The listing builds one solid part. Answer for the finished solid, in the listing's coordinates (mm). A direction names the side the tool comes from. Give positions to 0.01 mm unless a question says otherwise; leave off trailing zeros. Order: outer loops, then holes, each group sorted by start corner. A loop starts at its lowest first (then second) coordinate and runs counter-clockwise, first axis right, second up. Notation, with made-up numbers: (72.5, 66.25) - (120.5, 66.25) arc R15 ccw to (120.5, 81.25) - close; hole circle Ø6 at (-31, 51). An arc over 180 degrees is marked (long way). Answer in a Markdown table with one row per item.
from build123d import *

# Parameters (mm, degrees)
SKETCH1_R           = 2.5
SKETCH1_R_2         = 1.5
BOSS_EXTRUDE1_DEPTH = 55
SKETCH2_W           = 6
SKETCH2_H           = 1.5
BOSS_EXTRUDE2_DEPTH = 5
SKETCH3_R           = 1
CUT_EXTRUDE1_DEPTH  = 4.25
FILLET1_R           = 2


with BuildPart() as part:
    # Sketch1 → Boss-Extrude1 (new body)
    with BuildSketch(Plane(origin=(0, 0, 0), x_dir=(1, 0, 0), z_dir=(0, 1, 0))):
        Circle(SKETCH1_R)
        Circle(SKETCH1_R_2, mode=Mode.SUBTRACT)
    extrude(amount=BOSS_EXTRUDE1_DEPTH)

    # Sketch2 → Boss-Extrude2 (add)
    with BuildSketch(Plane(origin=(0, 55, 0), x_dir=(1, 0, 0), z_dir=(0, 1, 0))):
        Rectangle(SKETCH2_W, SKETCH2_H)
    extrude(amount=BOSS_EXTRUDE2_DEPTH)

    # Sketch3 → Cut-Extrude1 (cut, through all)
    with BuildSketch(Plane(origin=(0, 0, -0.75), x_dir=(-1, 0, 0), z_dir=(0, 0, -1))):
        with Locations((0, 58)):
            Circle(SKETCH3_R)
    extrude(amount=-CUT_EXTRUDE1_DEPTH, mode=Mode.SUBTRACT)

    # Fillet1
    fillet1_edges = [part.edges().sort_by_distance(p)[0] for p in [
        (3, 60, 0),
        (-3, 60, 0),
    ]]
    fillet(fillet1_edges, radius=FILLET1_R)


solid = part.part
Item 1: Find section A-A on x = 0. Write down the section's boundary in (y, z).
Answer block:
| item | result |
|---|---|
| outline | (0, -2.5) - (55, -2.5) - (55, -1.5) - (0, -1.5) - close; (0, 1.5) - (55, 1.5) - (55, 2.5) - (0, 2.5) - close; (55, -0.75) - (57, -0.75) - (57, 0.75) - (55, 0.75) - close; (59, -0.75) - (60, -0.75) - (60, 0.75) - (59, 0.75) - close |
Item 2: Find section B-B on z = 0. Write down the section's boundary in (x, y).
Answer block:
| item | result |
|---|---|
| outline | (-3, 55) - (-2.5, 55) - (-2.5, 0) - (-1.5, 0) - (-1.5, 55) - (1.5, 55) - (1.5, 0) - (2.5, 0) - (2.5, 55) - (3, 55) - (3, 58) arc R2 ccw to (1, 60) - (-1, 60) arc R2 ccw to (-3, 58) - close; hole circle Ø2 at (0, 58) |
Item 3: Each of these flat-tipped pins is pushed along its axis until it touches: P1, Ø1.5, axis at x = 1, y = 58.5, coming from the -Z side; P2, Ø1, axis at y = 14.5, z = -0.5, coming from the -X side; P3, Ø1.9, axis at x = 0, z = 2, coming from the +Y side. Where does it stop, or does it pass through?
Answer block:
| item | result |
|---|---|
| P1 | z = -0.75 |
| P2 | x = -2.5 |
| P3 | y = 55 |
Item 4: Find section C-C on y = 10.5. Write down the section's boundary in (x, z).
Answer block:
| item | result |
|---|---|
| outline | circle Ø5 at (0, 0); hole circle Ø3 at (0, 0) |
Item 5: Consider line 1 (Y direction, x = 0, z = 0.4); line 2 (Z direction, x = 0, y = 54). Determine where each line is inside the solid, lowest interval first.
Answer block:
| item | result |
|---|---|
| line 1 | 55 to 57, 59 to 60 |
| line 2 | -2.5 to -1.5, 1.5 to 2.5 |
Item 6: Determine the mould class of faces 5 (the face through (-0.54, 27.12, 2.44)), 6 (the face through (-2.43, 59.4, -0.01)), 7 (the face through (-0.54, 58.84, -0.01)), 8 (the face through (0, 0, 2)) for opening direction X: pulls with the +X half, pulls with the -X half, needs draft (parallel to the pull), parting line crosses it, or undercut.
Answer block:
| item | result |
|---|---|
| face 5 | parting line crosses it |
| face 6 | pulls with the -X half |
| face 7 | undercut |
| face 8 | needs draft |
Item 7: Which of the six approach directions +Z, -Z, +X, -X, +Y, -Y give full straight-line access (tool end or side, diameter ignored) to faces 1 (the face through (0, 55, 0)), 2 (the face through (0, 60, 0)), 3 (the face through (0, 55, -2)), 4 (the face through (1, 57, 0.75))?
Answer block:
| item | result |
|---|---|
| face 1 | -Y |
| face 2 | +Z, -Z, +X, -X, +Y |
| face 3 | -Z, +X, -X, +Y |
| face 4 | +Z, +X, -X, +Y |
